```python
from build123d import *

# Parameters (mm, degrees)
F0_W     = 91.6726738214
F0_H     = 44.5580258965
F0_W_2   = 80.7157829404
F0_H_2   = 35.7925109565
F1_DEPTH = 80
F2_START = 9
F0_R     = 10.8590602413
F2_DEPTH = 63
F3_R     = 5


with BuildPart() as f1:
    # F0 (on Top) → F1 (new body)
    with BuildSketch(Plane.XY):
        Rectangle(F0_W, F0_H)
        Rectangle(F0_W_2, F0_H_2, mode=Mode.SUBTRACT)
    extrude(amount=F1_DEPTH)

    # F0 (on Top) → F2 (join)
    with BuildSketch(Plane.XY.offset(F2_START)):
        Rectangle(F0_W_2, F0_H_2)
        with Locations((21.3659498841, 0)):
            Circle(F0_R, mode=Mode.SUBTRACT)
    extrude(amount=F2_DEPTH)

    # F3
    f3_edges = [f1.edges().sort_by_distance(p)[0] for p in [
        (45.836337, -22.279013, 40),
        (45.836337, 22.279013, 40),
        (-45.836337, 22.279013, 40),
        (-45.836337, -22.279013, 40),
    ]]
    fillet(f3_edges, radius=F3_R)


solid = f1.part
```
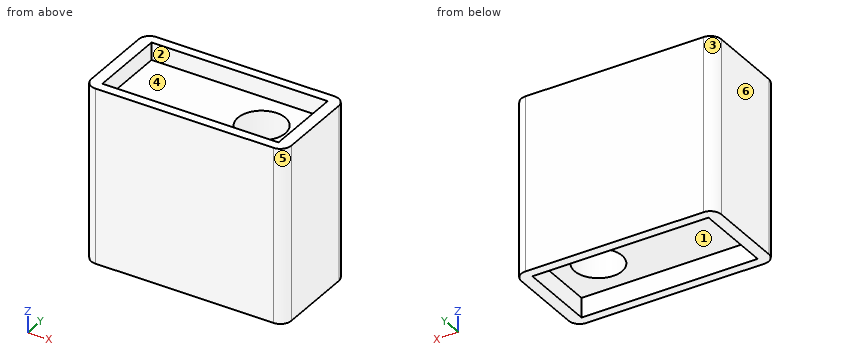
Can you work these out from the model? Positions are in its coordinate system, mm. Face numbers are marked on the shaded views. A direction names the side the tool comes from. Coordinates: 2 decimals unless noted, no trailing zeros. Loops run counter-clockwise (first coordinate to the right, second up) from the corner with the lowest first, then second, coordinate; pieces in that order, holes last. Notation, with made-up numbers: (26, 69.25) - (67, 69.25) arc R30 ccw to (67, 92.25) - close; hole circle Ø4 at (-18, 0.25). An arc over 180 degrees is marked (long way). Use a Markdown table: item, result.
Item 1: I want a section at A-A on z = 51.5. Please give me the cut outline in (x, y).
Numbers:
| item | result |
|---|---|
| outline | (-45.84, -17.28) arc R5 ccw to (-40.84, -22.28) - (40.84, -22.28) arc R5 ccw to (45.84, -17.28) - (45.84, 17.28) arc R5 ccw to (40.84, 22.28) - (-40.84, 22.28) arc R5 ccw to (-45.84, 17.28) - close; hole circle Ø21.72 at (21.37, 0) |
Item 2: If I drill on probe 1 along Y at (x, z) = (39.5, 75.5); probe 2 along Z at (x, y) = (14.5, -12); probe 3 along Y at (x, z) = (28, 45.5), over which ranges is the centre line in solid material (lowest first)? Write a range as from..to.
Numbers:
| item | result |
|---|---|
| probe 1 | y = -22.28..-17.9, 17.9..22.28 |
| probe 2 | z = 9..72 |
| probe 3 | y = -22.28..-8.6, 8.6..22.28 |
Item 3: For the marked faces 1, 2 and 3, which set-ups out of +Z, -Z, +X, -X, +Y, -Y let a thin tool reach every point of the face, with its end or its side?
Numbers:
| item | result |
|---|---|
| face 1 | -Z |
| face 2 | +Z |
| face 3 | +Z, -Z, -X, +Y |
Item 4: I want a section at C-C on y = -14. Please give me the cut outline in (x, z), and give its area (3 significant figures).
Numbers:
| item | result |
|---|---|
| outline | (-45.84, 0) - (-40.36, 0) - (-40.36, 9) - (40.36, 9) - (40.36, 0) - (45.84, 0) - (45.84, 80) - (40.36, 80) - (40.36, 72) - (-40.36, 72) - (-40.36, 80) - (-45.84, 80) - close |
| area | 5,960 mm2 |
Item 5: I want a section at D-D on x = -4.5. Please give me the cut outline in (y, z), and give its area (3 significant figures).
Numbers:
| item | result |
|---|---|
| outline | (-22.28, 0) - (-17.9, 0) - (-17.9, 9) - (17.9, 9) - (17.9, 0) - (22.28, 0) - (22.28, 80) - (17.9, 80) - (17.9, 72) - (-17.9, 72) - (-17.9, 80) - (-22.28, 80) - close |
| area | 2,960 mm2 |
Item 6: We'd pull the mould along Y, two halves only. Please class the marked faces 4, 5 and 6: released by +Y, released by -Y, zero draft, split by the parting line, or undercut.
Numbers:
| item | result |
|---|---|
| face 4 | undercut |
| face 5 | released by -Y |
| face 6 | zero draft |
Item 7: Will these pins go through, and if not, where does the flat tip stop? pin 1 (6 mm diameter, centred on x = -20.5, y = 11.5, fed in from -Z); pin 2 (13 mm diameter, centred on x = 21.37, y = 0, fed in from -Z) (3 decimals).
Numbers:
| item | result |
|---|---|
| pin 1 | stops at z = 9 |
| pin 2 | passes through |
Item 8: I want a section at B-B on y = 0. Please give me the cut outline in (x, z).
Numbers:
| item | result |
|---|---|
| outline | (-45.84, 0) - (-40.36, 0) - (-40.36, 9) - (10.51, 9) - (10.51, 72) - (-40.36, 72) - (-40.36, 80) - (-45.84, 80) - close; (32.23, 9) - (40.36, 9) - (40.36, 0) - (45.84, 0) - (45.84, 80) - (40.36, 80) - (40.36, 72) - (32.23, 72) - close |
